For this review, take the finished solid that the model builds, in its own axes (mm). Face numbers are marked on the shaded views. A direction names the side the tool comes from. Coordinates: 2 decimals unless noted, no trailing zeros. Order: outer loops, then holes, each group sorted by start corner. A loop starts at its lowest first (then second) coordinate and runs counter-clockwise, first axis right, second up. Notation, with made-up numbers: (31.25, -19.75) -> (37.25, -19.75) arc R17 cw to (37.25, 7.25) -> close; hole circle Ø4 at (-18.5, 87.25). An arc over 180 degrees is marked (long way). Write item = value, one per line. Start each with the question number.
1) Consider section C-C on x = 11. Give the boundary of the cut face in (y, z).
2) Consider section B-B on y = -0.5. Give the boundary of the cut face in (x, z).
3) Draft analysis for pull direction Y (two halves, no side actions). For the marked faces 5, 6 and 7, state which applies: +Y half, -Y half, draft (parallel to the pull), parting line (faces both ways), or undercut.
4) Wall thickness on probe 1 along Y at (x, z) = (11.75, 0.8); probe 2 along Y at (x, z) = (21, 0.5); probe 3 along X at (y, z) = (2.75, 0.55): over which ranges is each line inside the solid? List them lowest first. Write a range as [from, to].
5) Consider section A-A on z = 1.25. Give the boundary of the cut face in (x, y).
6) Consider section D-D on y = -3. Give the boundary of the cut face in (x, z), and give its area (3 significant figures).
7) Machinability: for the marked faces 1, 2, 3 and 4, which of the approach directions +Z, -Z, +X, -X, +Y, -Y give a long, thin tool a straight path to every point of the face, cutting with its end or side? Answer none if there is none.
8) Insertion check: pin 1 Ø3 at (x, y) = (23, -1) entering from -Z; pin 2 Ø0.5 at (x, z) = (8.5, 1) entering from -Y; pin 3 Ø0.5 at (x, z) = (12, 1) entering from -Y. Each pin has a flat end and moves straight along its axis. Give the tip position at first contact, or say it passes through.
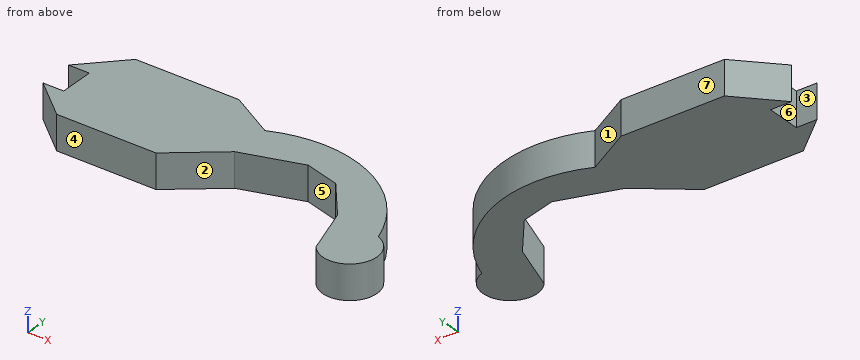
from build123d import *

# Parameters (mm, degrees)
BOSS_EXTRUDE1_DEPTH = 1.524


with BuildPart() as part:
    # Sketch1 → Boss-Extrude1 (new body)
    with BuildSketch(Plane.XY):
        with BuildLine():
            Line((8.880896155, 0), (7.962755207, 0))
            Line((7.962755207, 0), (9.635264959, -1.422689942))
            Line((9.635264959, -1.422689942), (14.039974044, -1.422689942))
            Line((14.039974044, -1.422689942), (16.231554776, 0.32393337))
            Line((16.231554776, 0.32393337), (18.872756066, 1.149856497))
            Line((18.872756066, 1.149856497), (20.404642344, 0.736894933))
            Line((20.404642344, 0.736894933), (21.744548774, -0.944356596))
            Line((21.744548774, -0.944356596), (22.435346644, -3.153443817))
            ThreePointArc((22.435346644, -3.153443817), (24.356473743, -3.107008643), (23.795164322, -1.269124727))
            ThreePointArc((23.795164322, -1.269124727), (20.773869568, 2.122690239), (16.231554776, 2.120028069))
            Line((16.231554776, 2.120028069), (14.223210267, 3.260079698))
            Line((14.223210267, 3.260079698), (9.635264959, 3.260079698))
            Line((9.635264959, 3.260079698), (7.962755207, 1.524))
            Line((7.962755207, 1.524), (8.880896155, 1.524))
            Line((8.880896155, 1.524), (8.880896155, 0))
        make_face()
    extrude(amount=BOSS_EXTRUDE1_DEPTH)


solid = part.part
Answer sheet:
q1.outline = (-1.42, 0) -> (3.26, 0) -> (3.26, 1.52) -> (-1.42, 1.52) -> close
q2.outline = (8.55, 0) -> (15.2, 0) -> (15.2, 1.52) -> (8.55, 1.52) -> close; (21.39, 0) -> (23.49, 0) -> (23.49, 1.52) -> (21.39, 1.52) -> close
q3.face_5 = -Y half
q3.face_6 = undercut
q3.face_7 = +Y half
q4.probe_1 = [-1.42, 3.26]
q4.probe_2 = [-0.01, 2.02]
q4.probe_3 = [9.14, 15.12]
q5.outline = (7.96, 0) -> (9.64, -1.42) -> (14.04, -1.42) -> (16.23, 0.32) -> (18.87, 1.15) -> (20.4, 0.74) -> (21.74, -0.94) -> (22.44, -3.15) arc R1.21 ccw (long way) to (23.8, -1.27) arc R5.55 ccw to (16.23, 2.12) -> (14.22, 3.26) -> (9.64, 3.26) -> (7.96, 1.52) -> (8.88, 1.52) -> (8.88, 0) -> close
q6.outline = (22.39, 0) -> (24.43, 0) -> (24.43, 1.52) -> (22.39, 1.52) -> close
q6.area = 3.11 mm2
q7.face_1 = +Z, -Z, +Y
q7.face_2 = +Z, -Z, -Y
q7.face_3 = +Z, -Z, -X
q7.face_4 = +Z, -Z, -X, -Y
q8.pin_1 = 0
q8.pin_2 = -0.67
q8.pin_3 = -1.42
